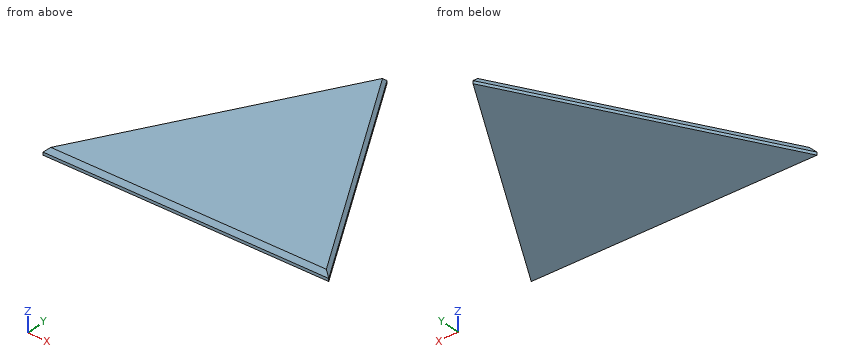
from build123d import *

# Parameters (mm, degrees)
F1_DEPTH = 8
F2_SIZE2 = 2.886751
F2_SIZE  = 5
F3_SIZE2 = 3.501038
F3_SIZE  = 5


with BuildPart() as f1:
    # F0 (on Top) → F1 (new body)
    with BuildSketch(Plane.XY):
        Polygon((-150, 0), (150, 0), (0, 259.807621), align=None)
    extrude(amount=F1_DEPTH)

    # F2
    f2_edges = [f1.edges().sort_by_distance(p)[0] for p in [
        (-75, 129.903811, 8),
        (75, 129.903811, 8),
    ]]
    chamfer(f2_edges, length=F2_SIZE, length2=F2_SIZE2)

    # F3
    f3_edges = [f1.edges().sort_by_distance(p)[0] for p in [
        (0, 0, 8),
    ]]
    chamfer(f3_edges, length=F3_SIZE, length2=F3_SIZE2)


solid = f1.part
Model file for the job. Use its own axes, mm. Give positions to 0.01 mm unless a question says otherwise; leave off trailing zeros. Order: outer loops, then holes, each group sorted by start corner. A loop starts at its lowest first (then second) coordinate and runs counter-clockwise, first axis right, second up. Notation, with made-up numbers: (70, 3.25) - (115, 3.25) arc R20 cw to (115, 28.25) - close; hole circle Ø7 at (-24, 9.5). An arc over 180 degrees is marked (long way). One line per item, written item: value.
Item 1: Slice it at A-A (x = -3.5). List the corners of the cut face in (y, z), then the cut area to 3 significant figures.
Response values:
outline: (0, 0) - (253.75, 0) - (253.75, 3) - (247.97, 8) - (3.5, 8) - (0, 3) - close
area: 2,010 mm2
Item 2: Wall check: line 1 (X direction, y = 172, z = 6); line 2 (X direction, y = 123.5, z = 4.5); line 3 (Y direction, x = -46, z = 1.5). Give the ranges that are in metal, low to high.
Response values:
line 1: -48.7 to 48.7
line 2: -77.7 to 77.7
line 3: 0 to 180.13
Item 3: Slice it at C-C (z = 6.75). List the corners of the cut face in (x, y), then the cut area to 3 significant figures.
Response values:
outline: (-145.98, 2.63) - (145.98, 2.63) - (0, 255.48) - close
area: 36,900 mm2
Item 4: Pin check, flat tips, straight feed: pin 1 Ø2 at (y, z) = (68, 5) entering from -X; pin 2 Ø4 at (y, z) = (74.5, 4.5) entering from +X; pin 3 Ø4 at (y, z) = (58.5, 6.5) entering from -X. Stop position of each tip, or through.
Response values:
pin 1: x = -110.29
pin 2: x = 107.75
pin 3: x = -115.66
Item 5: Slice it at B-B (y = 44.5). List the corners of the cut face in (x, z).
Response values:
outline: (-124.31, 0) - (124.31, 0) - (124.31, 3) - (120.97, 8) - (-120.97, 8) - (-124.31, 3) - close
